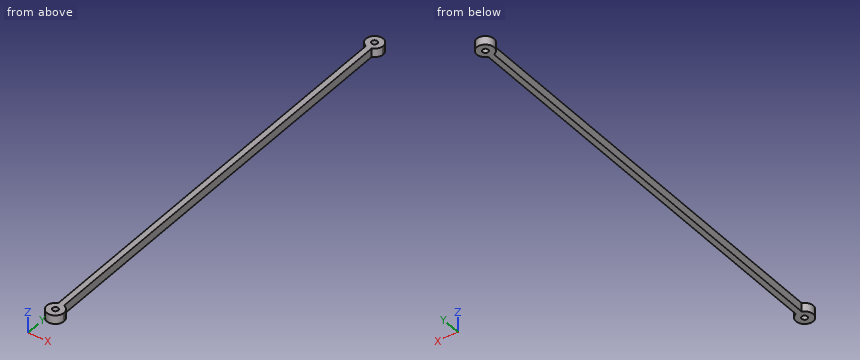
from build123d import *

# Parameters (mm, degrees)
EXTRUDE_3_DEPTH     = 3
SKETCH_3_R          = 1
CUT_EXTRUDE_1_DEPTH = 3


with BuildPart() as part:
    # Sketch 1 → Extrude 3 (new body)
    with BuildSketch(Plane.XY):
        with BuildLine():
            ThreePointArc((3, 0), (2.449489743, 1.732050808), (1, 2.828427125))
            Line((1, 2.828427125), (-1, 2.828427125))
            ThreePointArc((-1, 2.828427125), (-1.732050808, -2.449489743), (3, 0))
        make_face()
        with BuildLine():
            Line((-1, 2.828427125), (1, 2.828427125))
            ThreePointArc((1, 2.828427125), (0, 3), (-1, 2.828427125))
        make_face()
        with BuildLine():
            ThreePointArc((-1, 2.828427125), (0, 3), (1, 2.828427125))
            Line((1, 2.828427125), (1, 152.828427125))
            ThreePointArc((1, 152.828427125), (0, 152.656854249), (-1, 152.828427125))
            Line((-1, 152.828427125), (-1, 2.828427125))
        make_face()
        with BuildLine():
            ThreePointArc((-1, 152.828427125), (0, 152.656854249), (1, 152.828427125))
            Line((1, 152.828427125), (0, 152.828427125))
            Line((0, 152.828427125), (-1, 152.828427125))
        make_face()
        with BuildLine():
            Line((0, 152.828427125), (1, 152.828427125))
            ThreePointArc((1, 152.828427125), (2.449489743, 153.924803442), (3, 155.656854249))
            ThreePointArc((3, 155.656854249), (-1.732050808, 158.106343992), (-1, 152.828427125))
            Line((-1, 152.828427125), (0, 152.828427125))
        make_face()
    extrude(amount=EXTRUDE_3_DEPTH)

    # Sketch 3 → Cut-Extrude 1 (cut)
    with BuildSketch(Plane.XY.offset(3)):
        Circle(SKETCH_3_R)
        with Locations((0, 155.656854249)):
            Circle(SKETCH_3_R)
    extrude(amount=-CUT_EXTRUDE_1_DEPTH, mode=Mode.SUBTRACT)


solid = part.part
Work out the finished part from the listing and answer in its coordinate system (mm). Give positions to 0.01 mm unless a question says otherwise; leave off trailing zeros. Write each loop counter-clockwise with the first axis right and the second up, starting at its lowest first coordinate (ties: lowest second). Pieces come first, ordered by that corner, then holes.
Q1. Straight lines are drawn through the part: L1, parallel to Y at x = 0, z = 1.05; L2, parallel to Y at x = -0.75, z = 1.85; L3, parallel to X at y = 77.5, z = 1.95. For each, find the intervals that lie inside material, in ascending order.
Answer:
L1: y = -3 to -1, 1 to 154.66, 156.66 to 158.66
L2: y = -2.9 to -0.66, 0.66 to 155, 156.32 to 158.56
L3: x = -1 to 1
Q2. The part is cut by section A-A on x = 0. Give the vertices of the cut face in (y, z), and give its area (3 significant figures).
Answer:
outline: (-3, 0) - (-1, 0) - (-1, 3) - (-3, 3) - close; (1, 0) - (154.66, 0) - (154.66, 3) - (1, 3) - close; (156.66, 0) - (158.66, 0) - (158.66, 3) - (156.66, 3) - close
area: 473 mm2
Q3. The part is cut by section C-C on y = 25. Give the vertices of the cut face in (x, z), and give its area (3 significant figures).
Answer:
outline: (-1, 0) - (1, 0) - (1, 3) - (-1, 3) - close
area: 6.00 mm2
Q4. Given pin 1 (1.2 mm diameter, centred on x = 0, y = 155.66, fed in from +Z); pin 2 (1.5 mm diameter, centred on y = 115, z = 2, fed in from +X); pin 3 (1.5 mm diameter, centred on y = 50.5, z = 1, fed in from -X), each flat-ended and moving along its own axis, determine where each tip first touches the part or whether it passes through.
Answer:
pin 1: passes through
pin 2: stops at x = 1
pin 3: stops at x = -1
Q5. The part is cut by section B-B on z = 2.15. Give the vertices of the cut face in (x, y), and give its area (3 significant figures).
Answer:
outline: (-1, 2.83) arc R3 ccw (long way) to (1, 2.83) - (1, 152.83) arc R3 ccw (long way) to (-1, 152.83) - close; hole circle Ø2 at (0, 0); hole circle Ø2 at (0, 155.66)
area: 350 mm2
